```python
from build123d import *

# Parameters (mm, degrees)
CYLINDER035_R     = 1.75
CYLINDER035_DEPTH = 10
CYLINDER036_R     = 1.75
CYLINDER036_DEPTH = 10
CYLINDER033_R     = 200
CYLINDER033_DEPTH = 36
CYLINDER031_R     = 200
CYLINDER031_DEPTH = 53
BOX008_W          = 60
BOX008_H          = 99
BOX008_DEPTH      = 29
CYLINDER032_R     = 310
CYLINDER032_DEPTH = 77
CYLINDER030_R     = 700
CYLINDER030_DEPTH = 36
CYLINDER034_R     = 700
CYLINDER034_DEPTH = 36
FILLET006_R       = 4.2
BOX004_W          = 25
BOX004_H          = 10
BOX004_DEPTH      = 5


with BuildPart() as cylinder035:
    # Cylinder035 → Cylinder035 (new body)
    with BuildSketch(Plane(origin=(7.5, -47.5, 0), x_dir=(1, 0, 0), z_dir=(0, 0, 1))):
        Circle(CYLINDER035_R)
    extrude(amount=CYLINDER035_DEPTH)


with BuildPart() as screw_holes001:
    # Cylinder036 → Cylinder036 (new body)
    with BuildSketch(Plane(origin=(-7.5, -47.5, 0), x_dir=(1, 0, 0), z_dir=(0, 0, 1))):
        Circle(CYLINDER036_R)
    extrude(amount=CYLINDER036_DEPTH)

    # Fusion001: union Cylinder035
    add(cylinder035.part)


with BuildPart() as screw_holes001_1:
    # Fusion001 placement: moved
    add(screw_holes001.part.moved(Location((0, -1, 1))))


with BuildPart() as short_side_circle018:
    # Cylinder033 → Cylinder033 (new body)
    with BuildSketch(Plane(origin=(0, -154.8, 0), x_dir=(1, 0, 0), z_dir=(0, 0, 1))):
        Circle(CYLINDER033_R)
    extrude(amount=CYLINDER033_DEPTH)


with BuildPart() as short_side_circle016:
    # Cylinder031 → Cylinder031 (new body)
    with BuildSketch(Plane(origin=(1, 154.8, 0), x_dir=(1, 0, 0), z_dir=(0, 0, 1))):
        Circle(CYLINDER031_R)
    extrude(amount=CYLINDER031_DEPTH)


with BuildPart() as common028:
    # Box008 → Box008 (new body)
    with BuildSketch(Plane(origin=(-29.77, -50.31, 14), x_dir=(1, 0, 0), z_dir=(0, 0, 1))):
        with Locations((30, 49.5)):
            Rectangle(BOX008_W, BOX008_H)
    extrude(amount=BOX008_DEPTH)

    # Common028: intersect Short side circle016
    add(short_side_circle016.part, mode=Mode.INTERSECT)


with BuildPart() as common029:
    # Cylinder032 → Cylinder032 (new body)
    with BuildSketch(Plane(origin=(-32, 1, -262.75), x_dir=(0, 0, -1), z_dir=(1, 0, 0))):
        Circle(CYLINDER032_R)
    extrude(amount=CYLINDER032_DEPTH)

    # Common029: intersect Common028
    add(common028.part, mode=Mode.INTERSECT)


with BuildPart() as common030:
    # Cylinder030 → Cylinder030 (new body)
    with BuildSketch(Plane(origin=(671.8, 0, 0), x_dir=(1, 0, 0), z_dir=(0, 0, 1))):
        Circle(CYLINDER030_R)
    extrude(amount=CYLINDER030_DEPTH)

    # Common030: intersect Common029
    add(common029.part, mode=Mode.INTERSECT)


with BuildPart() as pad_cut002:
    # Cylinder034 → Cylinder034 (new body)
    with BuildSketch(Plane(origin=(-671.8, 0, 0), x_dir=(1, 0, 0), z_dir=(0, 0, 1))):
        Circle(CYLINDER034_R)
    extrude(amount=CYLINDER034_DEPTH)

    # Common031: intersect Common030
    add(common030.part, mode=Mode.INTERSECT)

    # Common032: intersect Short side circle018
    add(short_side_circle018.part, mode=Mode.INTERSECT)

    # Fillet006
    fillet006_edges = [pad_cut002.edges().sort_by_distance(p)[0] for p in [
        (26.845655, -43.522974, 25),
        (26.85399, 43.388958, 25),
        (-26.862626, -43.249676, 25),
        (-26.85399, 43.388958, 25),
    ]]
    fillet(fillet006_edges, radius=FILLET006_R)


with BuildPart() as pad_cut002_1:
    # Fillet006 placement: moved
    add(pad_cut002.part.moved(Location((0, 0, -15))))


with BuildPart() as obj1:
    # Box004 → Box004 (new body)
    with BuildSketch(Plane(origin=(-12.5, -53, 4), x_dir=(1, 0, 0), z_dir=(0, 0, 1))):
        with Locations((12.5, 5)):
            Rectangle(BOX004_W, BOX004_H)
    extrude(amount=BOX004_DEPTH)

    # Cut006: cut Pad cut002
    add(pad_cut002_1.part, mode=Mode.SUBTRACT)

    # Cut007: cut Screw holes001
    add(screw_holes001_1.part, mode=Mode.SUBTRACT)


solid = obj1.part
```
Here's how the part is built. I have some questions about the finished solid (model axes, mm). Coordinates: 2 decimals unless noted, no trailing zeros. Write each loop counter-clockwise with the first axis right and the second up, starting at its lowest first coordinate (ties: lowest second). Pieces come first, ordered by that corner, then holes. Notation, with made-up numbers: M -32.5,20 L 17.5,20 A30 cw 17.5,59 Z; hole C -6,71.25 d6. An arc over 180 degrees is marked long. Answer as CSV lines item,"result". Start each with the question number.
Q1. Suppose I cut it at D-D, the plane x = -7.5. List the corners of the cut face in (y, z) for me, then the cut area to 3 significant figures.
Q2. If we mould it in two halves opening along Y, with no side actions, what happens to faces 1 (the cylindrical face through (7.12, -50.21, 6.46)), 2 (the cylindrical face through (-7.88, -50.21, 6.46)), 3 (the flat face through (-12.5, -49, 6)), 4 (the cylindrical face through (-0.177, -45.197, 6.465))? For each: pulls with the +Y half, pulls with the -Y half, needs draft (parallel to the pull), parting line crosses it, or undercut.
Q3. I need wall thicknesses on probe 1 along X at (y, z) = (-48.5, 5.2); probe 2 along Y at (x, z) = (0.5, 7.15); probe 3 along Y at (x, z) = (7.5, 5.75). Which ranges of each line are inside material? Lowest first, please. Write a range as [from, to].
Q4. Suppose I cut it at A-A, the plane y = -48.5. List the corners of the cut face in (x, z) for me.
Q5. Suppose I cut it at B-B, the plane z = 4.55. List the corners of the cut face in (x, y) for me.
Q6. Suppose I cut it at C-C, the plane x = 9. List the corners of the cut face in (y, z) for me.
Entries:
1,outline,"M -53,4 L -50.25,4 L -50.25,9 L -53,9 Z; M -46.75,4 L -45.02,4 L -45.02,9 L -46.75,9 Z"
1,area,"22.4 mm²"
2,face 1,"undercut"
2,face 2,"undercut"
2,face 3,"needs draft"
2,face 4,"pulls with the +Y half"
3,probe 1,"x = [-12.5, -9.25], [-5.75, 5.75], [9.25, 12.5]"
3,probe 2,"y = [-53, -45.2]"
3,probe 3,"y = [-53, -50.25], [-46.75, -45.09]"
4,outline,"M -12.5,4 L -9.25,4 L -9.25,9 L -12.5,9 Z; M -5.75,4 L 5.75,4 L 5.75,9 L -5.75,9 Z; M 9.25,4 L 12.5,4 L 12.5,9 L 9.25,9 Z"
5,outline,"M -12.5,-53 L 12.5,-53 L 12.5,-44.87 A200 cw -12.5,-44.74 Z; hole C -7.5,-48.5 d3.5; hole C 7.5,-48.5 d3.5"
6,outline,"M -53,4 L -49.4,4 L -49.4,9 L -53,9 Z; M -47.6,4 L -45.04,4 L -45.04,9 L -47.6,9 Z"
